Check sheet for the modelled part. Datum: model origin and axes. Units: mm. A direction names the side the tool comes from. Round coordinates to 2 decimals unless told otherwise and drop trailing zeros. Loops run counter-clockwise (first coordinate to the right, second up) from the corner with the lowest first, then second, coordinate; pieces in that order, holes last. Notation, with made-up numbers: (43, 28.5) - (81, 28.5) arc R25 cw to (81, 65.5) - close; hole circle Ø5 at (70.25, -12). An arc over 180 degrees is marked (long way). Put each result on its own line as item: value. Start each with the question number.
```python
from build123d import *

# Parameters (mm, degrees)
SKETCH1_W           = 76.2
SKETCH1_H           = 50.8
BOSS_EXTRUDE1_DEPTH = 5.08
FILLET1_R           = 5.08
BOSS_EXTRUDE2_DEPTH = 5.08


with BuildPart() as part:
    # Sketch1 → Boss-Extrude1 (new body)
    with BuildSketch(Plane(origin=(0, 0, 0), x_dir=(1, 0, 0), z_dir=(0, 1, 0))):
        Rectangle(SKETCH1_W, SKETCH1_H)
    extrude(amount=BOSS_EXTRUDE1_DEPTH)

    # Fillet1
    fillet1_edges = [part.edges().sort_by_distance(p)[0] for p in [
        (38.1, 2.54, -25.4),
        (38.1, 2.54, 25.4),
        (-38.1, 2.54, 25.4),
        (-38.1, 2.54, -25.4),
    ]]
    fillet(fillet1_edges, radius=FILLET1_R)

    # Sketch2 → Boss-Extrude2 (add)
    with BuildSketch(Plane(origin=(0, 5.08, 0), x_dir=(1, 0, 0), z_dir=(0, 1, 0))):
        with BuildLine():
            Line((2.794, 10.190953103), (2.54, 13.605741995))
            ThreePointArc((2.54, 13.605741995), (13.840802551, 0), (2.54, -13.605741995))
            Line((2.54, -13.605741995), (2.794, -10.190953103))
            ThreePointArc((2.794, -10.190953103), (10.567022341, 0), (2.794, 10.190953103))
        make_face()
        with BuildLine():
            Line((-2.794, 10.190953103), (-2.54, 13.605741995))
            ThreePointArc((-2.54, 13.605741995), (-13.840802551, 0), (-2.54, -13.605741995))
            Line((-2.54, -13.605741995), (-2.794, -10.190953103))
            ThreePointArc((-2.794, -10.190953103), (-10.567022341, 0), (-2.794, 10.190953103))
        make_face()
    extrude(amount=BOSS_EXTRUDE2_DEPTH)


solid = part.part
```
Q1. Draft check along X on faces 5 (the face through (2.665, 7.584, 11.922)), 6 (the face through (36.651, 2.576, -23.872)), 7 (the face through (-11, 10.16, 0)). Enter one of: +X half, -X half, draft (parallel to the pull), parting line (faces both ways), or undercut.
Q2. Cross-section at D-D on x = -5. Enter the section's corners in (y, z).
Q3. Depth check by flat-ended pin: pin 1 Ø4 at (x, z) = (28, -19.5) entering from +Y; pin 2 Ø10 at (x, z) = (19, 3) entering from -Y. Enter the tip coordinate at first touch or a pass-through.
Q4. Cross-section at B-B on x = 12. Enter the section's corners in (y, z), and give its area (3 significant figures).
Q5. Cross-section at C-C on z = 3. Enter the section's corners in (x, y).
Q6. Cross-section at A-A on y = 6.75. Enter the section's corners in (x, z).
Q7. Material ranges on line 1 (Y direction, x = 4, z = 22.5); line 2 (Z direction, x = -4.5, y = 7); line 3 (X direction, y = 7, z = -6.5), recorded low to high. Write a range as from..to.
Q8. Set-up check for faces 1 (the face through (13.84, 7.58, -0.27)), 2 (the face through (-2.665, 7.584, 11.922)), 3 (the face through (36.572, 2.576, 23.951)), 4 (the face through (-13.84, 7.58, -0.27)): record each of +Z, -Z, +X, -X, +Y, -Y from which the full face is reachable in a straight line by a thin tool's end or side.
Answer list:
1. face 5: undercut
1. face 6: +X half
1. face 7: draft
2. outline: (0, -25.4) - (5.08, -25.4) - (5.08, -12.91) - (10.16, -12.91) - (10.16, -9.31) - (5.08, -9.31) - (5.08, 9.31) - (10.16, 9.31) - (10.16, 12.91) - (5.08, 12.91) - (5.08, 25.4) - (0, 25.4) - close
3. pin 1: stops at y = 5.08
3. pin 2: stops at y = 0
4. outline: (0, -25.4) - (5.08, -25.4) - (5.08, -6.9) - (10.16, -6.9) - (10.16, 6.9) - (5.08, 6.9) - (5.08, 25.4) - (0, 25.4) - close
4. area: 328 mm2
5. outline: (-38.1, 0) - (38.1, 0) - (38.1, 5.08) - (13.51, 5.08) - (13.51, 10.16) - (10.13, 10.16) - (10.13, 5.08) - (-10.13, 5.08) - (-10.13, 10.16) - (-13.51, 10.16) - (-13.51, 5.08) - (-38.1, 5.08) - close
6. outline: (-2.79, -10.19) arc R10.57 cw to (-2.79, 10.19) - (-2.54, 13.61) arc R13.84 ccw to (-2.54, -13.61) - close; (2.54, -13.61) arc R13.84 ccw to (2.54, 13.61) - (2.79, 10.19) arc R10.57 cw to (2.79, -10.19) - close
7. line 1: y = 0..5.08
7. line 2: z = -13.09..-9.56, 9.56..13.09
7. line 3: x = -12.22..-8.33, 8.33..12.22
8. face 1: +X, +Y
8. face 2: +Y
8. face 3: +Z, +X, +Y, -Y
8. face 4: -X, +Y
